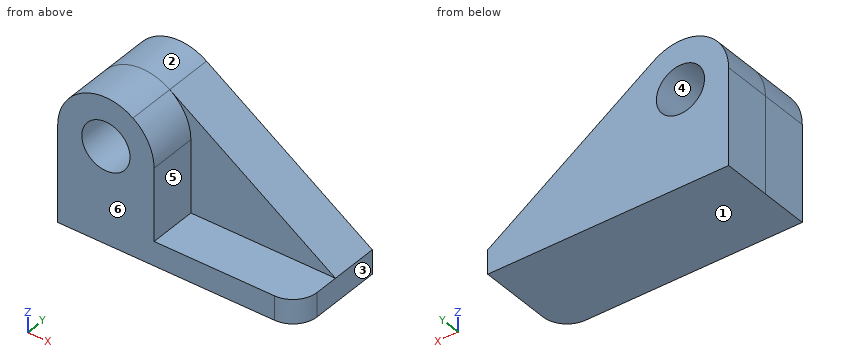
```python
from build123d import *

# Parameters (mm, degrees)
F0_R     = 12.7
F1_DEPTH = 25.4
F2_R     = 12.7
F3_DEPTH = 25.4
F4_R     = 12.7


# Not quite as in the source:
# - ends of sketch curves that miss each other by under 0.0002 mm in the source are joined


with BuildPart() as f1:
    # F0 (on Front) → F1 (new body)
    with BuildSketch(Plane.XZ):
        with BuildLine():
            Line((63.2129007654, 12.7), (-24.1528646808, 71.8148155579))
            ThreePointArc((-24.1528646808, 71.8148155579), (-50.2855998854, 73.2187510696), (-63.7870992346, 50.8))
            ThreePointArc((-63.7870992346, 50.8), (-63.78710636, 50.7890156001), (-63.7871087352, 50.7780311981))
            Line((-63.7871087352, 50.7780311981), (-63.7870992346, 0))
            Line((-63.7870992346, 0), (63.2129007654, 0))
            Line((63.2129007654, 0), (63.2129007654, 12.7))
        make_face()
        with Locations((-38.3871087352, 50.7780311981)):
            Circle(F0_R, mode=Mode.SUBTRACT)
    extrude(amount=F1_DEPTH)

    # F2 (on face) → F3 (join)
    with BuildSketch(Plane.XZ.offset(25.4)):
        with BuildLine():
            Line((-12.9871182357, 12.7), (-12.9871182357, 50.7780311981))
            ThreePointArc((-12.9871182357, 50.7780311981), (-15.951544937, 62.6862214229), (-24.1528700049, 71.8148076894))
            ThreePointArc((-24.1528700049, 71.8148076894), (-50.2855954349, 73.2187426759), (-63.7870897341, 50.7999999918))
            ThreePointArc((-63.7870897341, 50.7999999918), (-63.7870968595, 50.789015596), (-63.7870992346, 50.7780311981))
            Line((-63.7870992346, 50.7780311981), (-63.7870992346, 12.7))
            Line((-63.7870992346, 12.7), (-63.7870992346, 0))
            Line((-63.7870992346, 0), (63.2129007654, 0))
            Line((63.2129007654, 0), (63.2129007654, 12.7))
            Line((63.2129007654, 12.7), (-12.9871182357, 12.7))
        make_face()
        with Locations((-38.3871087352, 50.7780311981)):
            Circle(F2_R, mode=Mode.SUBTRACT)
    extrude(amount=F3_DEPTH)

    # F4
    f4_edges = [f1.edges().sort_by_distance(p)[0] for p in [
        (63.212901, -50.8, 6.35),
    ]]
    fillet(f4_edges, radius=F4_R)


solid = f1.part
```
CAD build for the part. Positions are in the model's coordinates, mm. Face numbers are marked on the shaded views. A direction names the side the tool comes from. Coordinates: 2 decimals unless noted, no trailing zeros.
(1) Drill centre lines: L1, parallel to Y at x = -11.5, z = 32; L2, parallel to Z at x = 41.5, y = -47.5; L3, parallel to Z at x = -30.5, y = -12. Where is each one in solid material? Low to high.
Solution:
L1: y = -25.4 to 0
L2: z = 0 to 12.7
L3: z = 0 to 40.82, 60.73 to 74.92
(2) Mould opens along X. For the marked faces 1, 2, 3 and 4 say: released by +X, released by -X, zero draft, split by the parting line, or undercut.
Solution:
face 1: zero draft
face 2: split by the parting line
face 3: released by +X
face 4: undercut
(3) Pin check, flat tips, straight feed: pin 1 Ø20.5 at (y, z) = (-38, 37) entering from +X; pin 2 Ø23 at (x, z) = (16, 28) entering from -Y; pin 3 Ø12.5 at (x, y) = (42.5, -39.5) entering from +Z. Stop position of each tip, or through.
Solution:
pin 1: stops at x = -12.99
pin 2: stops at y = -25.4
pin 3: stops at z = 12.7
(4) Which spindle directions (+Z, -Z, +X, -X, +Y, -Y) get a long thin tool onto all of the face, cutting with end or side? Do the marked faces 5 and 6. Say none if no direction does.
Solution:
face 5: +Z, +X, -Y
face 6: +Z, -Z, +X, -X, -Y
